```python
from build123d import *

# Parameters (mm, degrees)
F0_R     = 1.5875
F1_DEPTH = 3.175
F3_DEPTH = 1.5875
F5_DEPTH = 15.875
F6_W     = 5.5154263973
F6_H     = 0.8426345885
F7_DEPTH = 7.9375
F8_W     = 0.5498970859
F8_H     = 2.8869584203
F9_DEPTH = 12.7


# Not quite as in the source:
# - a feature names something its author has since deleted; it is built from what else it names


with BuildPart() as f1:
    # F0 (on Front) → F1 (new body)
    with BuildSketch(Plane.XZ):
        with BuildLine():
            ThreePointArc((16.3714576415, 16.2581077061), (15.790628657, 17.019159057), (14.8778171338, 17.3078398343))
            Line((14.8778171338, 17.3078398343), (-14.8778171338, 17.3078398343))
            ThreePointArc((-14.8778171338, 17.3078398343), (-15.790628657, 17.019159057), (-16.3714576415, 16.2581077061))
            Line((-16.3714576415, 16.2581077061), (-22.225, 0))
            Line((-22.225, 0), (-16.3714576415, -16.2581077061))
            ThreePointArc((-16.3714576415, -16.2581077061), (-15.790628657, -17.019159057), (-14.8778171338, -17.3078398343))
            Line((-14.8778171338, -17.3078398343), (14.8778171338, -17.3078398343))
            ThreePointArc((14.8778171338, -17.3078398343), (15.790628657, -17.019159057), (16.3714576415, -16.2581077061))
            Line((16.3714576415, -16.2581077061), (22.225, 0))
            Line((22.225, 0), (16.3714576415, 16.2581077061))
        make_face()
        with Locations((-18.0848, 0)):
            Circle(F0_R, mode=Mode.SUBTRACT)
        with BuildLine():
            ThreePointArc((-14.4999964, 14.1328398343), (-14.0350284151, 15.2553718495), (-12.9124964, 15.7203398343))
            Line((-12.9124964, 15.7203398343), (12.9124964, 15.7203398343))
            ThreePointArc((12.9124964, 15.7203398343), (14.0350284151, 15.2553718495), (14.4999964, 14.1328398343))
            Line((14.4999964, 14.1328398343), (14.4999964, -14.1328398343))
            ThreePointArc((14.4999964, -14.1328398343), (14.0350284151, -15.2553718495), (12.9124964, -15.7203398343))
            Line((12.9124964, -15.7203398343), (-12.9124964, -15.7203398343))
            ThreePointArc((-12.9124964, -15.7203398343), (-14.0350284151, -15.2553718495), (-14.4999964, -14.1328398343))
            Line((-14.4999964, -14.1328398343), (-14.4999964, 14.1328398343))
        make_face(mode=Mode.SUBTRACT)
        with Locations((18.0848, 0)):
            Circle(F0_R, mode=Mode.SUBTRACT)
        with BuildLine():
            Line((12.9124964, 15.7203398343), (-12.9124964, 15.7203398343))
            ThreePointArc((-12.9124964, 15.7203398343), (-14.0350284151, 15.2553718495), (-14.4999964, 14.1328398343))
            Line((-14.4999964, 14.1328398343), (-14.4999964, -14.1328398343))
            ThreePointArc((-14.4999964, -14.1328398343), (-14.0350284151, -15.2553718495), (-12.9124964, -15.7203398343))
            Line((-12.9124964, -15.7203398343), (12.9124964, -15.7203398343))
            ThreePointArc((12.9124964, -15.7203398343), (14.0350284151, -15.2553718495), (14.4999964, -14.1328398343))
            Line((14.4999964, -14.1328398343), (14.4999964, 14.1328398343))
            ThreePointArc((14.4999964, 14.1328398343), (14.0350284151, 15.2553718495), (12.9124964, 15.7203398343))
        make_face()
    extrude(amount=F1_DEPTH)

    # F2 (on face) → F3 (join)
    with BuildSketch(Plane.XZ.offset(3.175)):
        with BuildLine():
            Line((12.9124964, 15.7203398343), (-12.9124964, 15.7203398343))
            ThreePointArc((-12.9124964, 15.7203398343), (-14.0350284151, 15.2553718495), (-14.4999964, 14.1328398343))
            Line((-14.4999964, 14.1328398343), (-14.4999964, -14.1328398343))
            ThreePointArc((-14.4999964, -14.1328398343), (-14.0350284151, -15.2553718495), (-12.9124964, -15.7203398343))
            Line((-12.9124964, -15.7203398343), (12.9124964, -15.7203398343))
            ThreePointArc((12.9124964, -15.7203398343), (14.0350284151, -15.2553718495), (14.4999964, -14.1328398343))
            Line((14.4999964, -14.1328398343), (14.4999964, 14.1328398343))
            ThreePointArc((14.4999964, 14.1328398343), (14.0350284151, 15.2553718495), (12.9124964, 15.7203398343))
        make_face()
    extrude(amount=F3_DEPTH)

    # F4 (on face) → F5 (join)
    with BuildSketch(Plane(origin=(0, 0, 0), x_dir=(-1, 0, 0), z_dir=(0, 1, 0))):
        Polygon((6.35, 15.8496), (-6.35, 15.8496), (-14.5034, 7.9629), (-14.5034, -15.8496), (14.5034, -15.8496), (14.5034, 7.9629), align=None)
    extrude(amount=F5_DEPTH)

    # F6 (on face) → F7 (join)
    with BuildSketch(Plane(origin=(0, 15.875, 0), x_dir=(-1, 0, 0), z_dir=(0, 1, 0))):
        with Locations((0.0007232884, 13.041603379)):
            Rectangle(F6_W, F6_H)
        with Locations((-9.964916273, -0.3249486908)):
            Rectangle(F6_W, F6_H)
        with Locations((-9.8044754704, -12.5053403899)):
            Rectangle(F6_W, F6_H)
    extrude(amount=F7_DEPTH)

    # F8 (on face) → F9 (cut)
    with BuildSketch(Plane.XZ.offset(4.7625)):
        Polygon((-11.2841911614, 10.0093806594), (-11.2841911614, -1.6703880579), (11.2841911614, -1.6703880579), (11.2841911614, 10.0093806594), (7.5404811705, 12.8898254096), (-7.5404811705, 12.8898254096), align=None)
        with Locations((-7.3291899171, 6.8128034472)):
            Rectangle(F8_W, F8_H, mode=Mode.SUBTRACT)
        with Locations((7.0140829775, 6.8357163109)):
            Rectangle(F8_W, F8_H, mode=Mode.SUBTRACT)
        with Locations((0.0484438497, 9.8143247887)):
            Rectangle(F8_W, F8_H, mode=Mode.SUBTRACT)
    extrude(amount=-F9_DEPTH, mode=Mode.SUBTRACT)


solid = f1.part
```
The model under review builds one solid part; all positions refer to its coordinate system, in mm. A direction names the side the tool comes from. Round coordinates to 2 decimals unless told otherwise and drop trailing zeros. Loops run counter-clockwise (first coordinate to the right, second up) from the corner with the lowest first, then second, coordinate; pieces in that order, holes last.
Item 1: Take a section at A-A (y = 3.25). Write out the cut boundary in (x, z).
Determined:
outline: (-14.5, -15.85) - (14.5, -15.85) - (14.5, 7.96) - (6.35, 15.85) - (-6.35, 15.85) - (-14.5, 7.96) - close; (-7.6, 5.37) - (-7.05, 5.37) - (-7.05, 8.26) - (-7.6, 8.26) - close; (-0.23, 8.37) - (0.32, 8.37) - (0.32, 11.26) - (-0.23, 11.26) - close; (6.74, 5.39) - (7.29, 5.39) - (7.29, 8.28) - (6.74, 8.28) - close; hole (-11.28, -1.67) - (11.28, -1.67) - (11.28, 10.01) - (7.54, 12.89) - (-7.54, 12.89) - (-11.28, 10.01) - close
Item 2: Mouldability with a two-part tool opening along X and no side actions: class faces 5 (the face through (-15.802, -1.565, -17.011)), 6 (the face through (-7.604, 1, 7)), 7 (the face through (15, 0, 0)), 8 (the face through (14.02, -3.96, -15.27)) as released by +X, released by -X, zero draft, split by the parting line, or undercut.
Determined:
face 5: released by -X
face 6: undercut
face 7: zero draft
face 8: released by +X
Item 3: Take a section at B-B (x = 19). Write out the cut boundary in (y, z) (3 decimals), then the cut area to 3 significant figures.
Determined:
outline: (-3.175, -8.957) - (0, -8.957) - (0, -1.297) - (-3.175, -1.297) - close; (-3.175, 1.297) - (0, 1.297) - (0, 8.957) - (-3.175, 8.957) - close
area: 48.6 mm2
Item 4: Clearance check with flat-ended pins moving along their axes: pin 1 Ø6 at (x, z) = (17, 4.5) entering from +Y (3 decimals); pin 2 Ø2 at (x, y) = (8.5, 2.5) entering from +Z; pin 3 Ø0.9 at (y, z) = (0.5, 9) entering from +X. State where each tip first meets the part, or that it passes through.
Determined:
pin 1: stops at y = 15.875
pin 2: stops at z = 14.74
pin 3: stops at x = 13.9
Item 5: For faces 1 (the face through (9.44, 1.5, 11.43)), 2 (the face through (-10.484, 7.826, 11.851)), 3 (the face through (0, -4, 15.72)), 4 (the face through (10, 20, -0.746)), list the 3-axis set-ups (+Z, -Z, +X, -X, +Y, -Y) from which the entire face can be reached by the end or side of a thin tool; tool diameter is ignored.
Determined:
face 1: -Y
face 2: +Z, -X, +Y
face 3: +Z, +X, -X, -Y
face 4: +X, -X, +Y
Item 6: Take a section at C-C (y = 13). Write out the cut boundary in (x, z), then the cut area to 3 significant figures.
Determined:
outline: (-14.5, -15.85) - (14.5, -15.85) - (14.5, 7.96) - (6.35, 15.85) - (-6.35, 15.85) - (-14.5, 7.96) - close
area: 855 mm2
Item 7: Take a section at D-D (x = -4). Write out the cut boundary in (y, z) (1 decimal), then the cut area to 3 significant figures.
Determined:
outline: (-4.8, -15.7) - (-3.2, -15.7) - (-3.2, -17.3) - (0, -17.3) - (0, -15.8) - (15.9, -15.8) - (15.9, 15.8) - (0, 15.8) - (0, 17.3) - (-3.2, 17.3) - (-3.2, 15.7) - (-4.8, 15.7) - (-4.8, 12.9) - (7.9, 12.9) - (7.9, -1.7) - (-4.8, -1.7) - close
area: 478 mm2
Item 8: For line 1 (Z direction, x = 9.5, y = 19); line 2 (Z direction, x = 7, y = 6.75); line 3 (Y direction, x = -13, z = -15) (1 decimal), list the stretches that pass through material, from the lowest coordinate up.
Determined:
line 1: z = -12.93 to -12.08, -0.75 to 0.1
line 2: z = -15.85 to -1.67, 5.39 to 8.28, 12.89 to 15.22
line 3: y = -4.8 to 15.9
